Read the model definition and answer for the solid it produces. Units are mm, in the model's axes. Face numbers are marked on the shaded views. A direction names the side the tool comes from. Coordinates: 2 decimals unless noted, no trailing zeros. Write each loop counter-clockwise with the first axis right and the second up, starting at its lowest first coordinate (ties: lowest second). Pieces come first, ordered by that corner, then holes.
(1) Find the intervals of material crossed by probe 1 along Z at (x, y) = (-4.15, 0) (3 decimals); probe 2 along Y at (x, z) = (-4.25, -7.5); probe 3 along X at (y, z) = (6.5, 24), in increasing order.
(2) Which of the six approach directions +Z, -Z, +X, -X, +Y, -Y give full straight-line access (tool end or side, diameter ignored) to the marked faces 1 and 2?
(3) Given pin 1 (3 mm diameter, centred on x = -0.5, y = 37, fed in from -Z); pin 2 (2 mm diameter, centred on y = -45, z = 0, fed in from -X); pin 3 (3 mm diameter, centred on y = -2, z = -28.5, fed in from -X); pin 4 (5 mm diameter, centred on x = -9.5, z = 52, fed in from -Y), each flat-ended and moving along its own axis, determine where each tip first touches the part or whether it passes through.
(4) Section A-A on x = -9 is taken. Write down the section's boundary in (y, z).
(5) Section B-B on y = 38.5 is taken. State how many separate pieces and enclosed holes the cut face has, then the cut area to 3 significant figures.
(6) The mould has two halves that part along Z. Classify the marked faces 3 and 4: +Z half, -Z half, draft (parallel to the pull), parting line (faces both ways), or undercut.
Autodesk Inventor part; units mm, degrees
ref_plane "YZ Plane" through (0, 0, 0) normal (1, 0, 0) x (0, 1, 0)
ref_plane "XZ Plane" through (0, 0, 0) normal (0, 1, 0) x (-1, 0, 0)
ref_plane "XY Plane" through (0, 0, 0) normal (0, 0, 1) x (1, 0, 0)
sketch "Sketch1" plane through (0, 0, 0) normal (0, 1, 0) x (-1, 0, 0)
  line L0 (0, -96.425) -> (0, 8.05) construction
  line L1 (-6.1, 0) -> (15.6, 0) construction
  line L2 (-3, -8.5) -> (-3, -72.5)
  line L3 (1, -72.5) -> (12.5, -72.5)
  line L4 (12.5, -72.5) -> (12.5, -69.5777)
  line L5 (12.5, -69.5777) -> (5.5, -69.5777)
  line L6 (4.5, -23.5) -> (4.5, -8.5)
  line L7 (3, -8.5) -> (-3, -8.5)
  line L8 (4.5, -8.5) -> (4.5, -6.875)
  line L9 (4.5, -6.875) -> (3, -6.875)
  line L10 (3, -6.875) -> (3, -8.5)
  line L11 (5.5, -69.5777) -> (5.5, -67.5777)
  line L12 (5.5, -67.5777) -> (4.5, -67.5777)
  line L13 (4.5, -23.5) -> (0.5, -23.5)
  line L14 (0.5, -23.5) -> (0.5, -67.5777)
  line L15 (0.5, -67.5777) -> (4.5, -67.5777)
  line L16 (-3, -72.5) -> (-3, -81.5)
  line L17 (-3, -81.5) -> (1, -81.5)
  line L18 (1, -81.5) -> (1, -72.5)
  dimension "d6" = 69.5777
  dimension "d7" = 8.5
  dimension "d15" = 1.5
  dimension "d17" = 6
  dimension "d18" = 1.625
  dimension "d22" = 7
  dimension "d23" = 1
  dimension "d24" = 2
  dimension "d25" = 64
  dimension "d26" = 4
  dimension "d27" = 15
  dimension "d29" = 4
  dimension "d30" = 9
revolve "Revolution1" add sketch "Sketch1" angle 360 about axis through (0, 0, 0) along (-1, 0, 0)
chamfer "Chamfer1" distance 1 angle 45 2 edges at (3, 0, 8.5) (-12.5, 0, 69.5777)
sketch "Sketch2" plane through (-1, 0, 0) normal (-1, 0, 0) x (0, 0, 1)
  line L0 (0, 114.1) -> (0, -114.1) construction
  line L1 (-114.1, 0) -> (114.1, 0) construction
  circle A0 centre (0, 0) radius 77 construction
  circle A1 centre (0, 0) radius 72.5 construction
  circle A2 centre (0, 0) radius 81.5 construction
  point P0 (0, 77)
  dimension "d31" = 4.5
  dimension "d32" = 4.5
hole "Hole1" at (-1, 77, 0) direction (1, 0, 0) diameter 4.5 end through all
pattern_circular "Circular Pattern1" count 6 over 360 about axis through (-10, 0, 0) along (1, 0, 0) of "Hole1"
chamfer "Chamfer2" distance 0.4 angle 45 1 edges at (-12.5, 0, 72.5)
sketch "Sketch3" plane through (3, 0, 0) normal (1, 0, 0) x (0, 0, -1)
  line L0 (-114.1, 0) -> (114.1, 0) construction
  line L1 (0, -114.1) -> (0, 114.1) construction
  circle A0 centre (0, 0) radius 45 construction
  point P0 (0, 45)
  point P1 (-38.9711, 22.5)
  point P2 (-38.9711, -22.5)
  point P3 (0, -45)
  point P4 (38.9711, -22.5)
  point P5 (38.9711, 22.5)
  dimension "d46" = 90
  dimension "d49" = 360
hole "Hole2" at (3, 45, 0) at (3, 22.5, 38.9711) at (3, -22.5, 38.9711) at (3, -45, 0) at (3, -22.5, -38.9711) at (3, 22.5, -38.9711) direction (-1, 0, 0) diameter 2.459 depth 6.5 tip angle 118
equation "\"d6\" = 0.5 * D_ring"
equation "\"d31\" = d32"
equation "\"D_ring\" = D_ext"
properties part number "Housing_stage" material "Aluminum 6061"
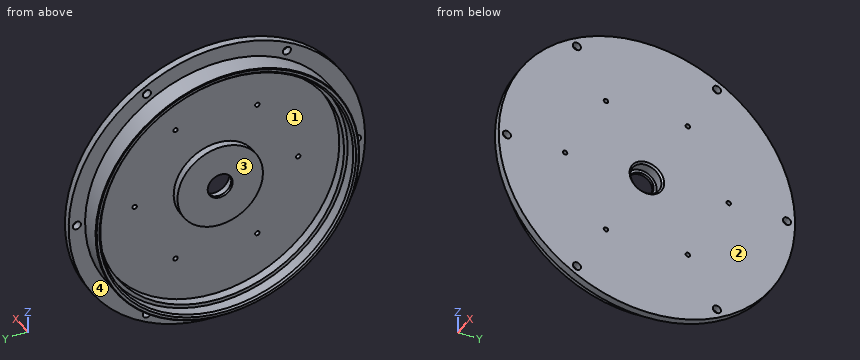
Response:
1. probe 1: z = -72.5 to -67.578, -23.5 to -6.875, 6.875 to 23.5, 67.578 to 72.5
1. probe 2: y = -72.11 to -67.16, -22.27 to 22.27, 67.16 to 72.11
1. probe 3: x = -0.5 to 3
2. face 1: -X
2. face 2: +Z, -Z, +X, +Y, -Y
3. pin 1: stops at z = -73.36
3. pin 2: passes through
3. pin 3: stops at x = -0.5
3. pin 4: stops at y = -52.97
4. outline: circle Ø145 at (0, 0); hole circle Ø139.16 at (0, 0)
5. separate pieces: 3
5. enclosed holes: 0
5. area: 583 mm2
6. face 3: undercut
6. face 4: draft
